```python
from build123d import *

# Parameters (mm, degrees)
SKETCH1_W                    = 82
SKETCH1_H                    = 50
SKETCH1_W_2                  = 23.5
SKETCH1_H_2                  = 15.6
BASE_FLANGE1_DEPTH           = 2
EDGE_FLANGE1_STRIP_W         = 9.4732
EDGE_FLANGE1_STRIP_H         = 2
EDGE_FLANGE1_STRIP_CUT_DEPTH = 82
EDGE_FLANGE1_DEPTH           = 82
EDGE_FLANGE2_STRIP_W         = 9.4732
EDGE_FLANGE2_STRIP_H         = 2
EDGE_FLANGE2_STRIP_CUT_DEPTH = 82
EDGE_FLANGE2_DEPTH           = 82
CUT_EXTRUDE1_DEPTH           = 153.144667997
CUT_EXTRUDE1_DEPTH_BACK      = 153.144667997
SKETCHED_START               = -63
SKETCHED_BEND2_OUTLINE_W     = 82
SKETCHED_BEND2_OUTLINE_H     = 50
SKETCHED_BEND2_DEPTH         = 63
SKETCHED_START_2             = -92
SKETCHED_BEND2_2_OUTLINE_W   = 26
SKETCHED_BEND2_2_OUTLINE_H   = 2
SKETCHED_BEND2_2_DEPTH       = 27
SKETCHED_START_3             = -62.2634
SKETCHED_BEND2_3_OUTLINE_W   = 82
SKETCHED_BEND2_3_OUTLINE_H   = 2
SKETCHED_BEND2_3_DEPTH       = 44.5268
SKETCHED_START_4             = -65
SKETCHED_BEND2_4_OUTLINE_W   = 26
SKETCHED_BEND2_4_OUTLINE_H   = 26.254644901
SKETCHED_BEND2_4_DEPTH       = 2
SKETCHED_BEND2_5_DEPTH       = 49
SKETCHED_BEND2_6_OUTLINE_W   = 2
SKETCHED_BEND2_6_OUTLINE_H   = 20
SKETCHED_BEND2_6_DEPTH       = 82
SKETCHED_BEND2_7_OUTLINE_W   = 2
SKETCHED_BEND2_7_OUTLINE_H   = 15.6
SKETCHED_BEND2_7_DEPTH       = 29.25
SKETCHED_START_5             = 52.75
SKETCHED_BEND2_8_OUTLINE_W   = 2
SKETCHED_BEND2_8_OUTLINE_H   = 15.6
SKETCHED_BEND2_8_DEPTH       = 29.25
SKETCHED_START_6             = 56
SKETCHED_BEND2_9_OUTLINE_W   = 2
SKETCHED_BEND2_9_OUTLINE_H   = 0.745355099
SKETCHED_BEND2_9_DEPTH       = 26
SKETCHED_START_7             = 29.25
SKETCHED_BEND2_10_DEPTH      = 19.75
FILLET1_R                    = 5
SKETCH19_R                   = 1.7
CUT_EXTRUDE2_DEPTH           = 10


with BuildPart() as part:
    # Base-Flange1: sheet metal written as solids
    # Sketch1 → Base-Flange1 (new body)
    with BuildSketch(Plane.XY):
        with Locations((41, -25)):
            Rectangle(SKETCH1_W, SKETCH1_H)
        with Locations((41, -27.8)):
            Rectangle(SKETCH1_W_2, SKETCH1_H_2, mode=Mode.SUBTRACT)
    extrude(amount=-BASE_FLANGE1_DEPTH)

    # Edge-Flange1: sheet metal written as solids
    # Edge-Flange1 strip (on a plane across the edge) → Edge-Flange1 strip cut (cut)
    with BuildSketch(Plane(origin=(82, -50, -2), x_dir=(0, 1, 0), z_dir=(-1, 0, 0))):
        with Locations((-2, -1)):
            Rectangle(EDGE_FLANGE1_STRIP_W, EDGE_FLANGE1_STRIP_H)
    extrude(amount=EDGE_FLANGE1_STRIP_CUT_DEPTH, mode=Mode.SUBTRACT)

    # Edge-Flange1 section (on a plane across the edge) → Edge-Flange1 (add)
    with BuildSketch(Plane(origin=(82, -50, -2), x_dir=(0, 1, 0), z_dir=(-1, 0, 0))):
        with BuildLine():
            Line((0, 0.7366), (0, 46))
            Line((0, 46), (2, 46))
            Line((2, 46), (2, 0.7366))
            ThreePointArc((2, 0.7366), (2.215745145, 0.215745145), (2.7366, 0))
            Line((2.7366, 0), (2.7366, -2))
            ThreePointArc((2.7366, -2), (0.801531583, -1.198468417), (0, 0.7366))
        make_face()
    extrude(amount=EDGE_FLANGE1_DEPTH)

    # Edge-Flange2: sheet metal written as solids
    # Edge-Flange2 strip (on a plane across the edge) → Edge-Flange2 strip cut (cut)
    with BuildSketch(Plane(origin=(0, -50, -48), x_dir=(0, 0, 1), z_dir=(1, 0, 0))):
        with Locations((-4, -1)):
            Rectangle(EDGE_FLANGE2_STRIP_W, EDGE_FLANGE2_STRIP_H)
    extrude(amount=EDGE_FLANGE2_STRIP_CUT_DEPTH, mode=Mode.SUBTRACT)

    # Edge-Flange2 section (on a plane across the edge) → Edge-Flange2 (add)
    with BuildSketch(Plane(origin=(0, -50, -48), x_dir=(0, 0, 1), z_dir=(1, 0, 0))):
        with BuildLine():
            Line((-2, 0.7366), (-2, 68))
            Line((-2, 68), (0, 68))
            Line((0, 68), (0, 0.7366))
            ThreePointArc((0, 0.7366), (0.215745145, 0.215745145), (0.7366, 0))
            Line((0.7366, 0), (0.7366, -2))
            ThreePointArc((0.7366, -2), (-1.198468417, -1.198468417), (-2, 0.7366))
        make_face()
    extrude(amount=EDGE_FLANGE2_DEPTH)

    # Sketch12 → Cut-Extrude1 (cut, two sides: drawn at the far end of the back side and taken through both)
    with BuildSketch(Plane(origin=(0, 0, -50), x_dir=(-1, 0, 0), z_dir=(0, 0, -1)).offset(-CUT_EXTRUDE1_DEPTH_BACK)):
        Polygon((-56, -92), (-82, -92), (-82, -118), (-49, -118), (-49, -63), (-56, -63), align=None)
        with BuildLine():
            Line((-75.25, -83.5), (-75.25, -81))
            ThreePointArc((-75.25, -81), (-77, -79.25), (-78.75, -81))
            Line((-78.75, -81), (-78.75, -83.5))
            ThreePointArc((-78.75, -83.5), (-77, -85.25), (-75.25, -83.5))
        make_face()
        with BuildLine():
            Line((-63.5, -83.5), (-63.5, -81))
            ThreePointArc((-63.5, -81), (-69, -75.5), (-74.5, -81))
            Line((-74.5, -81), (-74.5, -83.5))
            ThreePointArc((-74.5, -83.5), (-69, -89), (-63.5, -83.5))
        make_face()
        with BuildLine():
            Line((-44.25, -76), (-39.75, -76))
            ThreePointArc((-39.75, -76), (-36.75, -73), (-39.75, -70))
            Line((-39.75, -70), (-44.25, -70))
            ThreePointArc((-44.25, -70), (-47.25, -73), (-44.25, -76))
        make_face()
        with BuildLine():
            Line((-12.25, -76), (-7.75, -76))
            ThreePointArc((-7.75, -76), (-4.75, -73), (-7.75, -70))
            Line((-7.75, -70), (-12.25, -70))
            ThreePointArc((-12.25, -70), (-15.25, -73), (-12.25, -76))
        make_face()
        with BuildLine():
            Line((-12.25, -108), (-7.75, -108))
            ThreePointArc((-7.75, -108), (-4.75, -105), (-7.75, -102))
            Line((-7.75, -102), (-12.25, -102))
            ThreePointArc((-12.25, -102), (-15.25, -105), (-12.25, -108))
        make_face()
        with BuildLine():
            Line((-44.25, -108), (-39.75, -108))
            ThreePointArc((-39.75, -108), (-36.75, -105), (-39.75, -102))
            Line((-39.75, -102), (-44.25, -102))
            ThreePointArc((-44.25, -102), (-47.25, -105), (-44.25, -108))
        make_face()
        with BuildLine():
            ThreePointArc((-59.25, -81), (-61, -79.25), (-62.75, -81))
            Line((-62.75, -81), (-62.75, -83.5))
            ThreePointArc((-62.75, -83.5), (-61, -85.25), (-59.25, -83.5))
            Line((-59.25, -83.5), (-59.25, -81))
        make_face()
    extrude(amount=CUT_EXTRUDE1_DEPTH + CUT_EXTRUDE1_DEPTH_BACK, mode=Mode.SUBTRACT)

    # Sketched Bend2: read off the stored shape, not the designer's step
    # Sketched Bend2 outline → Sketched Bend2 (cut)
    with BuildSketch(Plane(origin=(0, 0, 0), x_dir=(1, 0, 0), z_dir=(0, 1, 0)).offset(SKETCHED_START)):
        with Locations((41, 25)):
            Rectangle(SKETCHED_BEND2_OUTLINE_W, SKETCHED_BEND2_OUTLINE_H)
    extrude(amount=SKETCHED_BEND2_DEPTH, mode=Mode.SUBTRACT)

    # Sketched Bend2 2 outline → Sketched Bend2 2 (cut)
    with BuildSketch(Plane(origin=(0, 0, 0), x_dir=(1, 0, 0), z_dir=(0, 1, 0)).offset(SKETCHED_START_2)):
        with Locations((69, 49)):
            Rectangle(SKETCHED_BEND2_2_OUTLINE_W, SKETCHED_BEND2_2_OUTLINE_H)
    extrude(amount=SKETCHED_BEND2_2_DEPTH, mode=Mode.SUBTRACT)

    # Sketched Bend2 4 outline → Sketched Bend2 4 (add)
    with BuildSketch(Plane(origin=(0, 0, 0), x_dir=(1, 0, 0), z_dir=(0, 1, 0)).offset(SKETCHED_START_4)):
        with Locations((69, 34.872677549)):
            Rectangle(SKETCHED_BEND2_4_OUTLINE_W, SKETCHED_BEND2_4_OUTLINE_H)
        with BuildLine():
            Line((59.25, 30.245355099), (59.25, 32.745355099))
            ThreePointArc((59.25, 32.745355099), (61, 34.495355099), (62.75, 32.745355099))
            Line((62.75, 32.745355099), (62.75, 30.245355099))
            ThreePointArc((62.75, 30.245355099), (61, 28.495355099), (59.25, 30.245355099))
        make_face(mode=Mode.SUBTRACT)
        with BuildLine():
            Line((63.5, 30.245355099), (63.5, 32.745355099))
            ThreePointArc((63.5, 32.745355099), (69, 38.245355099), (74.5, 32.745355099))
            Line((74.5, 32.745355099), (74.5, 30.245355099))
            ThreePointArc((74.5, 30.245355099), (69, 24.745355099), (63.5, 30.245355099))
        make_face(mode=Mode.SUBTRACT)
        with BuildLine():
            Line((75.25, 30.245355099), (75.25, 32.745355099))
            ThreePointArc((75.25, 32.745355099), (77, 34.495355099), (78.75, 32.745355099))
            Line((78.75, 32.745355099), (78.75, 30.245355099))
            ThreePointArc((78.75, 30.245355099), (77, 28.495355099), (75.25, 30.245355099))
        make_face(mode=Mode.SUBTRACT)
    extrude(amount=SKETCHED_BEND2_4_DEPTH)

    # Sketched Bend2 5 outline → Sketched Bend2 5 (cut)
    with BuildSketch(Plane.YZ):
        with BuildLine():
            ThreePointArc((-65.7366, -48), (-64.082332791, -48.556604688), (-63.100997602, -50))
            Line((-63.100997602, -50), (-63, -50))
            Line((-63, -50), (-63, -48))
            Line((-63, -48), (-65.7366, -48))
        make_face()
    extrude(amount=SKETCHED_BEND2_5_DEPTH, mode=Mode.SUBTRACT)



with BuildPart() as body_2:
    # Sketched Bend2 3 outline → Sketched Bend2 3 (new body)
    with BuildSketch(Plane(origin=(0, 0, 0), x_dir=(1, 0, 0), z_dir=(0, 1, 0)).offset(SKETCHED_START_3)):
        with Locations((41, 64.745355099)):
            Rectangle(SKETCHED_BEND2_3_OUTLINE_W, SKETCHED_BEND2_3_OUTLINE_H)
    extrude(amount=SKETCHED_BEND2_3_DEPTH)

    # Sketched Bend2 6 outline → Sketched Bend2 6 (add)
    with BuildSketch(Plane.YZ):
        with BuildLine():
            Line((-65, -50.745355099), (-65, -63.008755099))
            ThreePointArc((-65, -63.008755099), (-64.198468417, -64.943823516), (-62.2634, -65.745355099))
            Line((-62.2634, -65.745355099), (-62.2634, -63.745355099))
            ThreePointArc((-62.2634, -63.745355099), (-62.784254855, -63.529609954), (-63, -63.008755099))
            Line((-63, -63.008755099), (-63, -50.745355099))
            Line((-63, -50.745355099), (-65, -50.745355099))
        make_face()
        with Locations((-16, -103.745355099)):
            Rectangle(SKETCHED_BEND2_6_OUTLINE_W, SKETCHED_BEND2_6_OUTLINE_H)
        with BuildLine():
            Line((-17, -66.481955099), (-17, -78.145355099))
            Line((-17, -78.145355099), (-15, -78.145355099))
            Line((-15, -78.145355099), (-15, -66.481955099))
            ThreePointArc((-15, -66.481955099), (-15.801531582, -64.546886681), (-17.7366, -63.745355099))
            Line((-17.7366, -63.745355099), (-17.7366, -65.745355099))
            ThreePointArc((-17.7366, -65.745355099), (-17.215745145, -65.961100244), (-17, -66.481955099))
        make_face()
    extrude(amount=SKETCHED_BEND2_6_DEPTH)


with BuildPart() as part_1:
    add(part.part)

    add(body_2.part)  # Sketched Bend2 7 merges body 2
    # Sketched Bend2 7 outline → Sketched Bend2 7 (add)
    with BuildSketch(Plane.YZ):
        with BuildLine():
            Line((-65, -50.7366), (-65, -50.745355099))
            Line((-65, -50.745355099), (-63, -50.745355099))
            Line((-63, -50.745355099), (-63, -50.7366))
            ThreePointArc((-63, -50.7366), (-63.025366971, -50.364854094), (-63.100997602, -50))
            Line((-63.100997602, -50), (-65.7366, -50))
            ThreePointArc((-65.7366, -50), (-65.215745145, -50.215745145), (-65, -50.7366))
        make_face()
        with Locations((-16, -85.945355099)):
            Rectangle(SKETCHED_BEND2_7_OUTLINE_W, SKETCHED_BEND2_7_OUTLINE_H)
    extrude(amount=SKETCHED_BEND2_7_DEPTH)

    # Sketched Bend2 8 outline → Sketched Bend2 8 (add)
    with BuildSketch(Plane.YZ.offset(SKETCHED_START_5)):
        with Locations((-16, -85.945355099)):
            Rectangle(SKETCHED_BEND2_8_OUTLINE_W, SKETCHED_BEND2_8_OUTLINE_H)
    extrude(amount=SKETCHED_BEND2_8_DEPTH)

    # Sketched Bend2 9 outline → Sketched Bend2 9 (add)
    with BuildSketch(Plane.YZ.offset(SKETCHED_START_6)):
        with Locations((-64, -50.372677549)):
            Rectangle(SKETCHED_BEND2_9_OUTLINE_W, SKETCHED_BEND2_9_OUTLINE_H)
    extrude(amount=SKETCHED_BEND2_9_DEPTH)

    # Sketched Bend2 10 outline → Sketched Bend2 10 (add)
    with BuildSketch(Plane.YZ.offset(SKETCHED_START_7)):
        with BuildLine():
            Line((-65, -50.7366), (-65, -50.745355099))
            Line((-65, -50.745355099), (-63, -50.745355099))
            Line((-63, -50.745355099), (-63, -50.7366))
            ThreePointArc((-63, -50.7366), (-63.025366971, -50.364854094), (-63.100997602, -50))
            Line((-63.100997602, -50), (-65.7366, -50))
            ThreePointArc((-65.7366, -50), (-65.215745145, -50.215745145), (-65, -50.7366))
        make_face()
    extrude(amount=SKETCHED_BEND2_10_DEPTH)

    # Fillet1
    fillet1_edges = [part_1.edges().sort_by_distance(p)[0] for p in [
        (82, -64, -21.745355099),
        (56, -64, -21.745355099),
        (49, -118, -49),
        (0, -118, -49),
        (0, -16, -113.745355099),
        (82, -16, -113.745355099),
    ]]
    fillet(fillet1_edges, radius=FILLET1_R)

    # Sketch19 → Cut-Extrude2 (cut)
    with BuildSketch(Plane(origin=(0, 0, -65.745355099), x_dir=(-1, 0, 0), z_dir=(0, 0, -1))):
        with Locations(Location((-41, -32, 0), (0, 0, 90))):
            Circle(SKETCH19_R)
        with Locations(Location((-41, -55, 0), (0, 0, 90))):
            Circle(SKETCH19_R)
        with Locations(Location((-67, -31, 0), (0, 0, 90))):
            Circle(SKETCH19_R)
        with Locations(Location((-67, -49, 0), (0, 0, 90))):
            Circle(SKETCH19_R)
    extrude(amount=-CUT_EXTRUDE2_DEPTH, mode=Mode.SUBTRACT)


solid = part_1.part
```
The model under review builds one solid part; all positions refer to its coordinate system, in mm. A direction names the side the tool comes from. Round coordinates to 2 decimals unless told otherwise and drop trailing zeros. Order: outer loops, then holes, each group sorted by start corner. A loop starts at its lowest first (then second) coordinate and runs counter-clockwise, first axis right, second up.
(1) Mouldability with a two-part tool opening along X and no side actions: class faces 1 (the face through (15.25, -72.93, -48.99)), 2 (the face through (40, -40, -63.745)), 3 (the face through (80.496, -15.986, -112.32)) as released by +X, released by -X, zero draft, split by the parting line, or undercut.
Working result:
face 1: undercut
face 2: zero draft
face 3: released by +X
(2) Wall thickness on L1, parallel to X at y = -32, z = -65.05; L2, parallel to Y at x = 67, z = -64.6; L3, parallel to Y at x = 67, z = -64: over which ranges is each line inside the solid? List them lowest first.
Working result:
L1: x = 0 to 39.3, 42.7 to 65.63, 68.37 to 82
L2: y = -64.49 to -50.7, -47.3 to -32.7, -29.3 to -15.75
L3: y = -64.81 to -50.7, -47.3 to -32.7, -29.3 to -16.58
(3) Take a section at A-A, the plane y = -73. State the section outline as (x, z) points.
Working result:
outline: (0, -50) - (4.75, -50) - (4.75, -48) - (0, -48) - close; (15.25, -50) - (36.75, -50) - (36.75, -48) - (15.25, -48) - close; (47.25, -50) - (49, -50) - (49, -48) - (47.25, -48) - close
(4) Take a section at D-D, the plane y = -49. State the section outline as (x, z) points.
Working result:
outline: (0, -65.75) - (65.3, -65.75) - (65.3, -63.75) - (0, -63.75) - close; (68.7, -65.75) - (82, -65.75) - (82, -63.75) - (68.7, -63.75) - close
(5) Take a section at C-C, the plane z = -84.5. State the section outline as (x, y) points, plus the area to 3 significant figures.
Working result:
outline: (0, -17) - (29.25, -17) - (29.25, -15) - (0, -15) - close; (52.75, -17) - (82, -17) - (82, -15) - (52.75, -15) - close
area: 117 mm2
(6) Take a section at B-B, the plane x = 10. State the section outline as (y, z) points.
Working result:
outline: (-118, -50) - (-108, -50) - (-108, -48) - (-118, -48) - close; (-102, -50) - (-76, -50) - (-76, -48) - (-102, -48) - close; (-70, -50) - (-65.74, -50) arc R0.74 cw to (-65, -50.74) - (-65, -63.01) arc R2.74 ccw to (-62.26, -65.75) - (-17.74, -65.75) arc R0.74 cw to (-17, -66.48) - (-17, -113.75) - (-15, -113.75) - (-15, -66.48) arc R2.74 ccw to (-17.74, -63.75) - (-62.26, -63.75) arc R0.74 cw to (-63, -63.01) - (-63, -50.74) arc R2.74 ccw to (-65.74, -48) - (-70, -48) - close
(7) For P1, Ø2, axis at x = 39.5, y = -16.5, coming from the +Z side; P2, Ø1.6, axis at y = -64, z = -33.5, coming from the -X side; P3, Ø12, axis at x = 13.5, z = -40.5, coming from the -Y side; P4, Ø22.5, axis at x = 38, y = -35, coming from the -Z side, all flat-tipped, find the tip position at first contact; note any pin that passes through.
Working result:
P1: stops at z = -63.76
P2: stops at x = 56
P3: passes through
P4: stops at z = -65.75
(8) Tool access review of faces 4 (the face through (50, -63, -52)), 5 (the face through (40, -40, -65.745)), 6 (the face through (47.25, -72.93, -48.99)): name each direction out of +Z, -Z, +X, -X, +Y, -Y from which nothing blocks a thin tool from reaching the whole face with its end or side.
Working result:
face 4: +Z, +X, -X, +Y
face 5: -Z, +X, -X, -Y
face 6: +Z, -Z
